from build123d import *

# Parameters (mm, degrees)
BOSS_EXTRUDE1_DEPTH = 448.5
SKETCH2_R           = 4
CUT_EXTRUDE1_DEPTH  = 10
LPATTERN1_COUNT     = 3
LPATTERN1_PITCH     = 375


with BuildPart() as part:
    # Sketch1 → Boss-Extrude1 (new, symmetric)
    with BuildSketch(Plane.XY):
        Polygon((-18.924824174, 31.469740292), (-18.924824174, -13.530259708), (26.075175826, -13.530259708), (26.075175826, -18.530259708), (-23.924824174, -18.530259708), (-23.924824174, 31.469740292), align=None)
    extrude(amount=BOSS_EXTRUDE1_DEPTH, both=True)

    # Sketch2 → Cut-Extrude1 (cut)
    with BuildSketch(Plane.XZ.offset(18.530259708)):
        with Locations((6.075175826, 375)):
            Circle(SKETCH2_R)
    cut_extrude1 = extrude(amount=-CUT_EXTRUDE1_DEPTH, mode=Mode.SUBTRACT)

    # LPattern1: Cut-Extrude1 ×3
    with Locations(*[(0, 0, -i * LPATTERN1_PITCH) for i in range(1, LPATTERN1_COUNT)]):
        add(cut_extrude1, mode=Mode.SUBTRACT)


solid = part.part
Source: CAD feature listing. Evaluate the final solid. Frame: model axes, mm. A direction names the side the tool comes from. Round coordinates to 2 decimals unless told otherwise and drop trailing zeros. Write each loop counter-clockwise with the first axis right and the second up, starting at its lowest first coordinate (ties: lowest second). Pieces come first, ordered by that corner, then holes. Notation, with made-up numbers: M 73,58 L 111,58 A20 ccw 111,93 Z; hole C -9,29 d4. An arc over 180 degrees is marked long. One line per item, written item: value. Start each with the question number.
Item 1: Pin query (flat end, axial travel): pin 1 (8 mm diameter, centred on y = 22.5, z = -229, fed in from +X); pin 2 (13.5 mm diameter, centred on x = 9.5, z = 115, fed in from +Y). Return the tip coordinate at first contact, or that it passes through.
Item 2: Ray query, L1, parallel to X at y = -16.9, z = 375; L2, parallel to Y at x = 24, z = 378; L3, parallel to X at y = 8.5, z = -252.5. Return the intervals inside material, ascending. Write a range as from..to.
Item 3: Section query B-B (y = 20). Return the cut outline in (x, z), plus the area to 4 significant figures.
Item 4: Section query A-A (z = -113). Return the cut outline in (x, y).
Item 5: Set-up query: faces 1 (the flat face through (-10, -14, -448.5)), 2 (the flat face through (-18.925, 9, 6)). Return all of +Z, -Z, +X, -X, +Y, -Y with unobstructed straight access to the full face (end or side cutting, diameter ignored); none if empty.
Result set:
1. pin 1: stops at x = -18.92
1. pin 2: stops at y = -13.53
2. L1: x = -23.92..2.08, 10.08..26.08
2. L2: y = -18.53..-13.53
2. L3: x = -23.92..-18.92
3. outline: M -23.92,-448.5 L -18.92,-448.5 L -18.92,448.5 L -23.92,448.5 Z
3. area: 4,485 mm²
4. outline: M -23.92,-18.53 L 26.08,-18.53 L 26.08,-13.53 L -18.92,-13.53 L -18.92,31.47 L -23.92,31.47 Z
5. face 1: -Z, +X, -X, +Y, -Y
5. face 2: +Z, -Z, +X, +Y
